```python
from build123d import *

# Parameters (mm, degrees)
SKETCH1_W                  = 12
SKETCH1_H                  = 6
BOSS_EXTRUDE1_DEPTH        = 6
F_60_0_04_DIAMETER_HOLE1_D = 1.016
SKETCH15_W                 = 6
SKETCH15_H                 = 6
BOSS_EXTRUDE2_DEPTH        = 7
FILLET4_R                  = 0.5
FILLET3_R                  = 1.5
SKETCH19_R                 = 1.35
CUT_EXTRUDE1_DEPTH         = 5.5
SKETCH16_R                 = 1.35
CUT_EXTRUDE2_DEPTH         = 5


with BuildPart() as part:
    # Sketch1 → Boss-Extrude1 (new body)
    with BuildSketch(Plane(origin=(0, 0, 0), x_dir=(1, 0, 0), z_dir=(0, 1, 0))):
        Rectangle(SKETCH1_W, SKETCH1_H)
    extrude(amount=BOSS_EXTRUDE1_DEPTH)

    # 60 _0.04_ Diameter Hole1 (through all)
    with Locations(Plane(origin=(0, 6, 0), x_dir=(1, 0, 0), z_dir=(0, 1, 0))):
        with Locations((1.008, 0), (-1.008, 0)):
            Hole(F_60_0_04_DIAMETER_HOLE1_D / 2)

    # Sketch15 → Boss-Extrude2 (add)
    with BuildSketch(Plane.XY.offset(3)):
        with Locations((0, 3)):
            Rectangle(SKETCH15_W, SKETCH15_H)
    extrude(amount=BOSS_EXTRUDE2_DEPTH)

    # Fillet4
    fillet4_edges = [part.edges().sort_by_distance(p)[0] for p in [
        (-4.5, 6, 3),
        (4.5, 0, 3),
        (4.5, 6, 3),
        (-4.5, 0, 3),
        (0, 0, -3),
        (0, 6, -3),
    ]]
    fillet(fillet4_edges, radius=FILLET4_R)

    # Fillet3
    # the kernel refuses this fillet: 1.5 mm, written as the material it adds along each edge
    with BuildSketch(Plane(origin=(3, 0.5, 3), x_dir=(1, 0, 0), z_dir=(0, 1, 0)), Plane(origin=(-3, 5.5, 3), x_dir=(-1, 0, 0), z_dir=(0, -1, 0))) as fillet3_piece_1:
        with BuildLine():
            CenterArc((FILLET3_R, -FILLET3_R), FILLET3_R, 90, 90)
            Line((0, -FILLET3_R), (0, 0))
            Line((0, 0), (FILLET3_R, 0))
        make_face()
    extrude(amount=5)
    with BuildSketch(Plane(origin=(3, 0.5, 2.5), x_dir=(0, 0.006283143965558622, 0.9999802608561372), z_dir=(0, -0.9999802608561372, 0.006283143965558622))) as fillet3_piece_2_section:
        with BuildLine():
            CenterArc((-0.5 - FILLET3_R, -FILLET3_R), FILLET3_R, 0, 90)
            Line((-0.5 - FILLET3_R, 0), (-0.5, 0))
            Line((-0.5, 0), (-0.5, -FILLET3_R))
        make_face()
    fillet3_piece_2 = revolve(axis=Axis((3, 0.5, 2.5), (-1, 0, 0)), revolution_arc=359.64, mode=Mode.PRIVATE)
    fillet3_piece_2 = split(fillet3_piece_2, bisect_by=Plane(origin=(3.567816549, 0, 2.882028447), z_dir=(0, 1, 0)), keep=Keep.TOP, mode=Mode.PRIVATE)
    add(fillet3_piece_2)
    with BuildSketch(Plane(origin=(3, 5.5, 2.5), x_dir=(0, -0.0062831439655592885, 0.9999802608561372), z_dir=(0, 0.9999802608561372, 0.0062831439655592885))) as fillet3_piece_3_section:
        with BuildLine():
            CenterArc((-0.5 - FILLET3_R, FILLET3_R), FILLET3_R, 270, 90)
            Line((-0.5 - FILLET3_R, 0), (-0.5, 0))
            Line((-0.5, 0), (-0.5, FILLET3_R))
        make_face()
    fillet3_piece_3 = revolve(axis=Axis((3, 5.5, 2.5), (1, 0, 0)), revolution_arc=359.64, mode=Mode.PRIVATE)
    fillet3_piece_3 = split(fillet3_piece_3, bisect_by=Plane(origin=(3.567816573, 6, 2.8820284), z_dir=(0, -1, 0)), keep=Keep.TOP, mode=Mode.PRIVATE)
    add(fillet3_piece_3)
    with BuildSketch(Plane(origin=(-3, 0.5, 2.5), x_dir=(0, 0, 1), z_dir=(0, 1, 0))) as fillet3_piece_4_section:
        with BuildLine():
            CenterArc((0.5 + FILLET3_R, -FILLET3_R), FILLET3_R, 90, 90)
            Line((0.5 + FILLET3_R, 0), (0.5, 0))
            Line((0.5, 0), (0.5, -FILLET3_R))
        make_face()
    fillet3_piece_4 = revolve(axis=Axis((-3, 0.5, 2.5), (1, 0, 0)), revolution_arc=359.64, mode=Mode.PRIVATE)
    fillet3_piece_4 = split(fillet3_piece_4, bisect_by=Plane(origin=(-3.567816642, 0, 2.882028407), z_dir=(0, 1, 0)), keep=Keep.TOP, mode=Mode.PRIVATE)
    add(fillet3_piece_4)
    with BuildSketch(Plane(origin=(-3, 5.5, 2.5), x_dir=(0, 0, 1), z_dir=(0, -1, 0))) as fillet3_piece_5_section:
        with BuildLine():
            CenterArc((0.5 + FILLET3_R, FILLET3_R), FILLET3_R, 180, 90)
            Line((0.5 + FILLET3_R, 0), (0.5, 0))
            Line((0.5, 0), (0.5, FILLET3_R))
        make_face()
    fillet3_piece_5 = revolve(axis=Axis((-3, 5.5, 2.5), (-1, 0, 0)), revolution_arc=359.64, mode=Mode.PRIVATE)
    fillet3_piece_5 = split(fillet3_piece_5, bisect_by=Plane(origin=(-3.567816642, 6, 2.882028407), z_dir=(0, -1, 0)), keep=Keep.TOP, mode=Mode.PRIVATE)
    add(fillet3_piece_5)

    # Sketch19 → Cut-Extrude1 (cut)
    with BuildSketch(Plane.ZY.offset(6)):
        with Locations((0, 3)):
            Circle(SKETCH19_R)
    cut_extrude1 = extrude(amount=-CUT_EXTRUDE1_DEPTH, mode=Mode.SUBTRACT)

    # Sketch16 → Cut-Extrude2 (cut)
    with BuildSketch(Plane.XY.offset(10)):
        with Locations((0, 3)):
            Circle(SKETCH16_R)
    extrude(amount=-CUT_EXTRUDE2_DEPTH, mode=Mode.SUBTRACT)

    # Mirror2: Cut-Extrude1 across plane
    add(cut_extrude1.mirror(Plane(origin=(0, 0, 0), x_dir=(0, 0, 1), z_dir=(1, 0, 0))), mode=Mode.SUBTRACT)


solid = part.part
```
Input: part model. Units: mm. Frame: model coordinates. A direction names the side the tool comes from. Give positions to 0.01 mm unless a question says otherwise; leave off trailing zeros. Order: outer loops, then holes, each group sorted by start corner. A loop starts at its lowest first (then second) coordinate and runs counter-clockwise, first axis right, second up.
1. Cut plane A-A (x = -2). Return loops of the section in (y, z).
Computed:
outline: (0, -2.5) arc R0.5 ccw to (0.5, -3) - (5.5, -3) arc R0.5 ccw to (6, -2.5) - (6, 10) - (0, 10) - close; hole circle Ø2.7 at (3, 0)
2. Line query: probe 1 along Y at (x, z) = (3.75, 0.5); probe 2 along Z at (x, y) = (-1, 1); probe 3 along Z at (x, y) = (2.8, 3). Output: solid intervals per line, ascending.
Computed:
probe 1: y = 0 to 1.75, 4.25 to 6
probe 2: z = -3 to -0.51, 0.51 to 10
probe 3: z = -3 to -1.35, 1.35 to 10
3. Pin query (flat end, axial travel): pin 1 Ø2.5 at (y, z) = (3, 0) entering from -X; pin 2 Ø1.2 at (x, y) = (-5, 4) entering from +Z; pin 3 Ø1.7 at (y, z) = (2, 6) entering from +X. Return the tip coordinate at first contact, or that it passes through.
Computed:
pin 1: stops at x = -0.5
pin 2: stops at z = 3
pin 3: stops at x = 3
4. Draft query along X for faces 1 (the face through (0, 3, 5)), 2 (the face through (3, 3, 7)), 3 (the face through (1.516, 0.862, -0.022)), 4 (the face through (-0.7, 4.4, 10)). Return one class per face: released by +X, released by -X, zero draft, split by the parting line, or undercut.
Computed:
face 1: undercut
face 2: released by +X
face 3: undercut
face 4: zero draft
5. Cut plane D-D (x = 0). Return loops of the section in (y, z), and give its area (3 significant figures).
Computed:
outline: (0, -2.5) arc R0.5 ccw to (0.5, -3) - (5.5, -3) arc R0.5 ccw to (6, -2.5) - (6, 10) - (4.35, 10) - (4.35, 5) - (1.65, 5) - (1.65, 10) - (0, 10) - close
area: 64.4 mm2
6. Cut plane B-B (y = 1.5). Return loops of the section in (x, z).
Computed:
outline: (-6, -3) - (6, -3) - (6, 3) - (4.5, 3) arc R1.5 cw to (3, 4.5) - (3, 10) - (-3, 10) - (-3, 4.5) arc R1.5 cw to (-4.5, 3) - (-6, 3) - close; hole circle Ø1.02 at (-1.01, 0); hole circle Ø1.02 at (1.01, 0)
7. Set-up query: faces 5 (the face through (-5, 3, 3)), 6 (the face through (-0.5, 3, 0)), 7 (the face through (5, 3, 3)), 8 (the face through (0.5, 3, 0)). Return all of +Z, -Z, +X, -X, +Y, -Y with unobstructed straight access to the full face (end or side cutting, diameter ignored); none if empty.
Computed:
face 5: +Z, -X, +Y, -Y
face 6: -X
face 7: +Z, +X, +Y, -Y
face 8: +X
8. Cut plane C-C (z = 7.75). Return loops of the section in (x, y).
Computed:
outline: (-3, 0) - (3, 0) - (3, 6) - (-3, 6) - close; hole circle Ø2.7 at (0, 3)
